Answer from the drawing. Dimensions are ordinates in mm from the lowest x, y and z of the part. A direction names the side the tool comes from. Give positions to 0.01 mm unless a question says otherwise; leave off trailing zeros. Write each loop counter-clockwise with the first axis right and the second up, starting at its lowest first coordinate (ties: lowest second). Pieces come first, ordered by that corner, then holes.
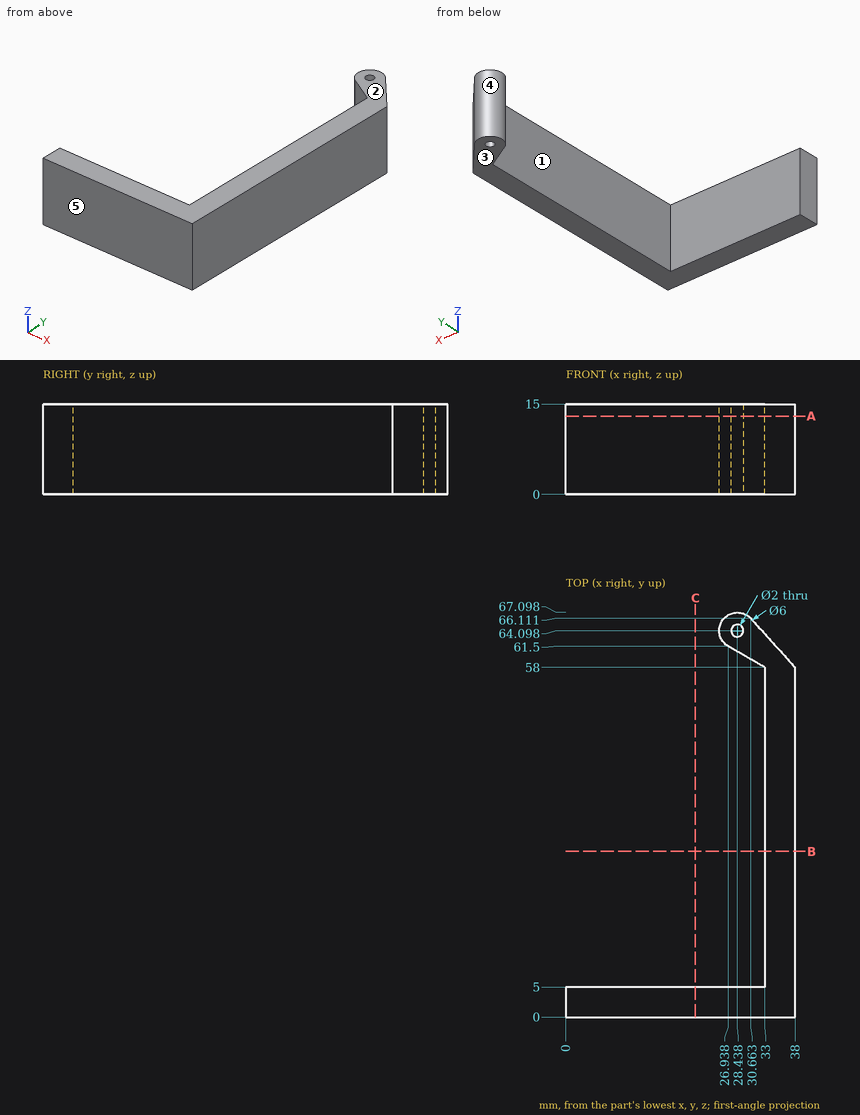
Item 1: Consider probe 1 along Y at (x, z) = (29, 2.25) (1 decimal); probe 2 along Y at (x, z) = (19.5, 14); probe 3 along X at (y, z) = (50, 7.25). Determine where each line is inside the solid, lowest interval first.
Conclusion:
probe 1: y = 0 to 5, 60.3 to 63.3, 64.9 to 67
probe 2: y = 0 to 5
probe 3: x = 33 to 38
Item 2: A cutting plane is placed at A-A, the plane z = 13. Give the vertices of the cut face in (x, y).
Conclusion:
outline: (0, 0) - (38, 0) - (38, 58) - (30.66, 66.11) arc R3 ccw (long way) to (26.94, 61.5) - (33, 58) - (33, 5) - (0, 5) - close; hole circle Ø2 at (28.44, 64.1)
Item 3: Determine the mould class of the marked faces 3, 4 and 5 for opening direction Y: pulls with the +Y half, pulls with the -Y half, needs draft (parallel to the pull), parting line crosses it, or undercut.
Conclusion:
face 3: needs draft
face 4: undercut
face 5: pulls with the -Y half
Item 4: A cutting plane is placed at B-B, the plane y = 27.5. Give the vertices of the cut face in (x, z).
Conclusion:
outline: (33, 0) - (38, 0) - (38, 15) - (33, 15) - close
Item 5: A cutting plane is placed at C-C, the plane x = 21.5. Give the vertices of the cut face in (y, z), plus the area to 3 significant figures.
Conclusion:
outline: (0, 0) - (5, 0) - (5, 15) - (0, 15) - close
area: 75.0 mm2
Item 6: Each of these flat-tipped pins is pushed along its axis until it touches: P1, Ø4.5, axis at x = 12.5, z = 9, coming from the +Y side; P2, Ø6, axis at y = 58, z = 11, coming from the -X side (1 decimal); P3, Ø5, axis at y = 55, z = 12, coming from the -X side. Where does it stop, or does it pass through?
Conclusion:
P1: stops at y = 5
P2: stops at x = 27.8
P3: stops at x = 33
Item 7: Which of the six approach directions +Z, -Z, +X, -X, +Y, -Y give full straight-line access (tool end or side, diameter ignored) to the marked faces 1 and 2?
Conclusion:
face 1: +Z, -Z, -X
face 2: +Z, +X, -X, +Y, -Y
